```python
from build123d import *

# Parameters (mm, degrees)
F1_DEPTH = 13
F4_W     = 39.5263805985
F4_H     = 30.6198559701
F5_DEPTH = 12
F3_W     = 39.7066194564
F3_H     = 27.9853120446
F6_DEPTH = 25


with BuildPart() as f1:
    # F0 (on Front) → F1 (new body)
    with BuildSketch(Plane.XZ):
        Polygon((75.2189680934, 76.4205157757), (-74.2607861757, 76.778665185), (-74.2607861757, -75.2398595214), (75.2189680934, -75.2398595214), align=None)
    extrude(amount=-F1_DEPTH)

    # F4 (on face) → F5 (join)
    with BuildSketch(Plane.XZ):
        with Locations((24.8862691224, 28.5907592624)):
            Rectangle(F4_W, F4_H)
    extrude(amount=-F5_DEPTH)

    # F3 (on face) → F6 (join)
    with BuildSketch(Plane(origin=(0, 13, 0), x_dir=(-1, 0, 0), z_dir=(0, 1, 0))):
        with Locations((27.4936407804, 30.1694050431)):
            Rectangle(F3_W, F3_H)
    extrude(amount=-F6_DEPTH)


solid = f1.part
```
The listing builds one solid part. Answer for the finished solid, in the listing's coordinates (mm). A direction names the side the tool comes from. Round coordinates to 2 decimals unless told otherwise and drop trailing zeros. Write each loop counter-clockwise with the first axis right and the second up, starting at its lowest first coordinate (ties: lowest second). Pieces come first, ordered by that corner, then holes. Notation, with made-up numbers: (70.5, -15.5) -> (118.5, -15.5) arc R31 cw to (118.5, 18.5) -> close; hole circle Ø9 at (58.25, -26.75). An arc over 180 degrees is marked (long way). Answer as a JSON object with one key per item and string values. Group by question number.
Q1. Section C-C (y = -7.5) is taken. Write down the section's boundary in (x, z).
Q2. Which of the six approach directions +Z, -Z, +X, -X, +Y, -Y give full straight-line access (tool end or side, diameter ignored) to faces 1 (the face through (-27, -6, 16.177)), 2 (the face through (-7.64, -6, 30)), 3 (the face through (-27, -6, 44.162)), 4 (the face through (-47.347, -6, 30)), 5 (the face through (2, 13, 2))?
Q3. Section A-A (z = 39.5) is taken. Write down the section's boundary in (x, y), plus the area to 3 significant figures.
Q4. Section B-B (x = -26) is taken. Write down the section's boundary in (y, z).
Q5. Straight lines are drawn through the part: line 1 along X through (y, z) = (-2, 34); line 2 along Y through (x, z) = (32, -53); line 3 along Z through (x, y) = (61.5, 2.25). For each, find the intervals that lie inside material, in ascending order.
Q6. Each of these flat-tipped pins is pushed along its axis until it touches: pin 1 Ø12 at (x, z) = (-42.5, -15.5) entering from -Y; pin 2 Ø13 at (x, y) = (-23.5, -8.5) entering from +Z; pin 3 Ø9.5 at (y, z) = (-8.5, 36) entering from +X. Where does it stop, or does it pass through?
Q7. Section D-D (z = -31) is taken. Write down the section's boundary in (x, y), plus the area to 3 significant figures.
Check values:
{
 "1": {"outline": "(-47.35, 16.18) -> (-7.64, 16.18) -> (-7.64, 44.16) -> (-47.35, 44.16) -> close"},
 "2": {"face 1": "-Z, +X, -X, -Y", "face 2": "+Z, -Z, +X, -Y", "face 3": "+Z, +X, -X, -Y", "face 4": "+Z, -Z, -X, -Y", "face 5": "+Z, -Z, +X, -X, +Y"},
 "3": {"outline": "(-74.26, 0) -> (-47.35, 0) -> (-47.35, -12) -> (-7.64, -12) -> (-7.64, 0) -> (75.22, 0) -> (75.22, 13) -> (-74.26, 13) -> close", "area": "2,420 mm^2"},
 "4": {"outline": "(-12, 16.18) -> (0, 16.18) -> (0, -75.24) -> (13, -75.24) -> (13, 76.66) -> (0, 76.66) -> (0, 44.16) -> (-12, 44.16) -> close"},
 "5": {"line 1": "-47.35 to -7.64", "line 2": "0 to 13", "line 3": "-75.24 to 76.45"},
 "6": {"pin 1": "y = 0", "pin 2": "z = 44.16", "pin 3": "x = -7.64"},
 "7": {"outline": "(-74.26, 0) -> (75.22, 0) -> (75.22, 13) -> (-74.26, 13) -> close", "area": "1,940 mm^2"}
}
